Can you work these out from the model? Positions are in its coordinate system, mm. Give positions to 0.01 mm unless a question says otherwise; leave off trailing zeros. Loops run counter-clockwise (first coordinate to the right, second up) from the corner with the lowest first, then second, coordinate; pieces in that order, holes last. Notation, with made-up numbers: (-18.75, 86.5) -> (5.25, 86.5) arc R10 ccw to (5.25, 102.5) -> close; hole circle Ø1 at (31.5, 51.5). An arc over 180 degrees is marked (long way). Use CSV: the item, a comma, the result in double quotes.
Autodesk Inventor part; units mm, degrees
ref_plane "YZ Plane" through (0, 0, 0) normal (1, 0, 0) x (0, 1, 0)
ref_plane "XZ Plane" through (0, 0, 0) normal (0, 1, 0) x (-1, 0, 0)
ref_plane "XY Plane" through (0, 0, 0) normal (0, 0, 1) x (1, 0, 0)
sketch "Esquisse12" plane through (0, 0, 0) normal (0, 0, 1) x (1, 0, 0)
  line L0 (0, 0) -> (20, 0)
  line L1 (20, 0) -> (20, 38)
  line L2 (20, 38) -> (0, 38)
  line L3 (0, 38) -> (0, 0)
  line L4 (10, 38) -> (10, 0) construction
  circle A0 centre (10, 7) radius 2.21
  line L5 (10, 7) -> (20, 7) construction
  circle A1 centre (16, 7) radius 2.21
  circle A2 centre (4, 7) radius 2.21
  circle A3 centre (10, 7) radius 2.21
  circle A4 centre (10, 25) radius 2.21
  circle A5 centre (16, 25) radius 2.21
  circle A6 centre (4, 25) radius 2.21
  dimension "d133" = 20
  dimension "d134" = 7
  dimension "d135" = 4.42
  dimension "d138" = 6
  dimension "d141" = 6
  dimension "d148" = 18
  dimension "d153" = 13
extrude "Extrusion13" add sketch "Esquisse12" along normal blind 2.2
fillet "Congé8" radius 7 2 edges at (20, 0, 1.1) (0, 0, 1.1)
mirror "Symétrie3" about plane through (20, 38, 0) normal (0, 1, 0)
equation "\"d135\" = Holes"
equation "\"d154\" = Depth"
equation "\"d156\" = Rounding"
equation "\"Depth\" = 2.2"
equation "\"Holes\" = 4.42"
equation "\"Height\" = 0"
equation "\"Rounding\" = 7"
properties part number "SideToSide"
(1) If we section it at B-B, the plane z = 1.65: Give the number of separate pieces and of enclosed holes in the cut face, then the cut area to 3 significant figures.
Answer sheet:
separate pieces,"1"
enclosed holes,"12"
area,"1,290 mm2"
(2) If I drill on L1, parallel to Y at x = 10, z = 0.45; L2, parallel to X at y = 69, z = 1.55; L3, parallel to Y at x = 16, z = 0.65, over which ranges is the centre line in solid material (lowest first)? Write a range as from..to.
Answer sheet:
L1,"y = 0..4.79, 9.21..22.79, 27.21..48.79, 53.21..66.79, 71.21..76"
L2,"x = 0..1.79, 6.21..7.79, 12.21..13.79, 18.21..20"
L3,"y = 0.68..4.79, 9.21..22.79, 27.21..48.79, 53.21..66.79, 71.21..75.32"
(3) If we section it at C-C, the plane x = 4.75: Write out the boundary of the cut face in (y, z).
Answer sheet:
outline,"(0.37, 0) -> (4.92, 0) -> (4.92, 2.2) -> (0.37, 2.2) -> close; (9.08, 0) -> (22.92, 0) -> (22.92, 2.2) -> (9.08, 2.2) -> close; (27.08, 0) -> (48.92, 0) -> (48.92, 2.2) -> (27.08, 2.2) -> close; (53.08, 0) -> (66.92, 0) -> (66.92, 2.2) -> (53.08, 2.2) -> close; (71.08, 0) -> (75.63, 0) -> (75.63, 2.2) -> (71.08, 2.2) -> close"
(4) We'd pull the mould along X, two halves only. Please class faces 1 (the face through (3.521, 9.157, 1.085)), 2 (the face through (10, 39, 2.2)), 3 (the face through (17.9, 2, 1.1)): released by +X, released by -X, zero draft, split by the parting line, or undercut.
Answer sheet:
face 1,"undercut"
face 2,"zero draft"
face 3,"released by +X"
(5) If we section it at A-A, the plane x = 10: Write out the boundary of the cut face in (y, z).
Answer sheet:
outline,"(0, 0) -> (4.79, 0) -> (4.79, 2.2) -> (0, 2.2) -> close; (9.21, 0) -> (22.79, 0) -> (22.79, 2.2) -> (9.21, 2.2) -> close; (27.21, 0) -> (48.79, 0) -> (48.79, 2.2) -> (27.21, 2.2) -> close; (53.21, 0) -> (66.79, 0) -> (66.79, 2.2) -> (53.21, 2.2) -> close; (71.21, 0) -> (76, 0) -> (76, 2.2) -> (71.21, 2.2) -> close"
(6) Will these pins go through, and if not, where does the flat tip stop? pin 1 Ø2.5 at (x, y) = (4, 25) entering from -Z; pin 2 Ø1 at (x, z) = (4.5, 0.5) entering from -Y.
Answer sheet:
pin 1,"passes through"
pin 2,"stops at y = 0.29"
